```python
from build123d import *

# Parameters (mm, degrees)
SKETCH_1_W        = 65.7
SKETCH_1_H        = 16
EXTRUDE_1_DEPTH   = 2
FILLET_1_R        = 0.5
HOLE_WIZARD_M31_D = 3.15


with BuildPart() as part:
    # Эскиз1 → Бобышка-Вытянуть1 (new body)
    with BuildSketch(Plane(origin=(0, 0, 0), x_dir=(1, 0, 0), z_dir=(0, 1, 0))):
        Rectangle(SKETCH_1_W, SKETCH_1_H)
    extrude(amount=-EXTRUDE_1_DEPTH)

    # Скругление1
    fillet_1_edges = [part.edges().sort_by_distance(p)[0] for p in [
        (32.85, -1, 8),
        (-32.85, -1, 8),
        (-32.85, -1, -8),
        (32.85, -1, -8),
    ]]
    fillet(fillet_1_edges, radius=FILLET_1_R)

    # Сверло под метчик  спиральное M31 (through all)
    with Locations(Plane(origin=(0, 0, 0), x_dir=(1, 0, 0), z_dir=(0, 1, 0))):
        with Locations((18.5, -4), (-18.5, -4)):
            Hole(HOLE_WIZARD_M31_D / 2)


solid = part.part
```
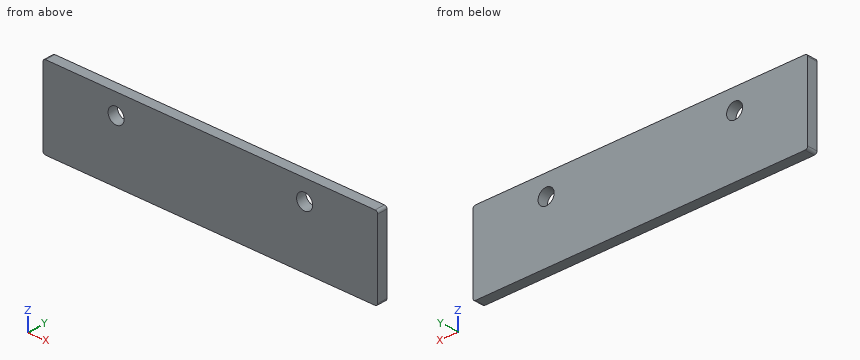
Can you work these out from the model? Positions are in its coordinate system, mm. Give positions to 0.01 mm unless a question says otherwise; leave off trailing zeros. Order: outer loops, then holes, each group sorted by start corner. A loop starts at its lowest first (then second) coordinate and runs counter-clockwise, first axis right, second up. Notation, with made-up numbers: M 77,-19 L 126,-19 A14 cw 126,-2 Z; hole C -20,26 d10. An arc over 180 degrees is marked long. One line per item, written item: value.
1) I want a section at A-A, the plane x = -18.5. List the corners of the cut face in (y, z) for me (3 decimals).
Answer sheet:
outline: M -2,-8 L 0,-8 L 0,2.425 L -2,2.425 Z; M -2,5.575 L 0,5.575 L 0,8 L -2,8 Z
2) Please list where these lines run through material, in increasing order: line 1 along X through (y, z) = (-0.85, 4) (3 decimals); line 2 along Z through (x, y) = (-18.5, -0.9) (3 decimals); line 3 along X through (y, z) = (-0.75, 5).
Answer sheet:
line 1: x = -32.85 to -20.075, -16.925 to 16.925, 20.075 to 32.85
line 2: z = -8 to 2.425, 5.575 to 8
line 3: x = -32.85 to -19.72, -17.28 to 17.28, 19.72 to 32.85
3) I want a section at B-B, the plane y = -0.75. List the corners of the cut face in (x, z) for me (3 decimals).
Answer sheet:
outline: M -32.85,-7.5 A0.5 ccw -32.35,-8 L 32.35,-8 A0.5 ccw 32.85,-7.5 L 32.85,7.5 A0.5 ccw 32.35,8 L -32.35,8 A0.5 ccw -32.85,7.5 Z; hole C -18.5,4 d3.15; hole C 18.5,4 d3.15
4) For P1, Ø5, axis at x = 18.5, z = 4, coming from the -Y side, with a flat end and sliding along its axis, tell me the tip position at first contact or that it passes through.
Answer sheet:
P1: stops at y = -2
5) I want a section at C-C, the plane z = 4. List the corners of the cut face in (x, y) for me (3 decimals), plus the area to 3 significant figures.
Answer sheet:
outline: M -32.85,-2 L -20.075,-2 L -20.075,0 L -32.85,0 Z; M -16.925,-2 L 16.925,-2 L 16.925,0 L -16.925,0 Z; M 20.075,-2 L 32.85,-2 L 32.85,0 L 20.075,0 Z
area: 119 mm^2
